Can you work these out from the model? Positions are in its coordinate system, mm. A direction names the side the tool comes from. Coordinates: 2 decimals unless noted, no trailing zeros. Order: outer loops, then holes, each group sorted by start corner. A loop starts at its lowest first (then second) coordinate and runs counter-clockwise, first axis right, second up. Notation, with made-up numbers: (78.25, 17.25) - (92.25, 17.25) arc R18 ccw to (92.25, 25.25) - close; hole circle Ø1 at (57.5, 9.5). An arc over 180 degrees is marked (long way). Use a Markdown table: item, result. Add a question column.
(1) I want a section at D-D (z = -5.5). List the corners of the cut face in (x, y) for me.
(2) I want a section at B-B (y = 0). List the corners of the cut face in (x, z) for me, and give its area (3 significant figures).
(3) We'd pull the mould along X, two halves only. Please class faces 1 (the cylindrical face through (-13.976, 14.868, 23.171)), 2 (the flat face through (-18.6, -18.7, 23.2)), 3 (the flat face through (3, 0, -2)): pulls with the +X half, pulls with the -X half, needs draft (parallel to the pull), parting line crosses it, or undercut.
(4) I want a section at A-A (z = 18). List the corners of the cut face in (x, y) for me, and give its area (3 significant figures).
(5) If I drill on L1, parallel to Y at x = -15.5, z = 29.5; L2, parallel to Z at x = 4, y = -8; L3, parallel to Z at x = -4, y = 11, over which ranges is the centre line in solid material (lowest first)? Write a range as [from, to].
(6) I want a section at C-C (x = 0). List the corners of the cut face in (y, z) for me, and give its area (3 significant figures).
(7) On a 3-axis mill with a long thin cutter (end or side, diameter ignored), from which of +Z, -Z, +X, -X, +Y, -Y can I reach the whole of each face in a straight line? I mean faces 4 (the cylindrical face through (17.024, 14.868, 23.171)), 5 (the cylindrical face through (-0.1, -2.5, -7.9)), 6 (the flat face through (0, 2, -8)). Say none if no direction works.
(8) For pin 1 Ø21 at (x, y) = (-3, -8) entering from -Z; pin 2 Ø0.9 at (x, z) = (0.5, -8) entering from +Y; pin 3 Ø3 at (x, z) = (-5, -4.5) entering from -Y; pin 4 Ø4 at (x, y) = (15.5, -15.5) entering from -Z, each with a flat end and sliding along its axis, tell me the tip position at first contact or that it passes through.
```python
from build123d import *

# Parameters (mm, degrees)
SKETCH_1_R          = 1.65
EXTRUDE_1_DEPTH     = 47
SKETCH_3_R          = 11
EXTRUDE_2_DEPTH     = 2
EXTRUDE_3_DEPTH     = 22
CUT_EXTRUDE_1_DEPTH = 10


with BuildPart() as part:
    # 草图1 → 凸台-拉伸1 (new body)
    with BuildSketch(Plane.XY):
        Polygon((-21.15, 16.15), (-16.15, 21.15), (16.15, 21.15), (21.15, 16.15), (21.15, -16.15), (16.15, -21.15), (-16.15, -21.15), (-21.15, -16.15), align=None)
        with Locations((15.5, 15.5)):
            Circle(SKETCH_1_R, mode=Mode.SUBTRACT)
        with Locations((-15.5, 15.5)):
            Circle(SKETCH_1_R, mode=Mode.SUBTRACT)
        with Locations((15.5, -15.5)):
            Circle(SKETCH_1_R, mode=Mode.SUBTRACT)
        with Locations((-15.5, -15.5)):
            Circle(SKETCH_1_R, mode=Mode.SUBTRACT)
    extrude(amount=EXTRUDE_1_DEPTH)

    # 草图3 → 凸台-拉伸2 (add)
    with BuildSketch(Plane(origin=(0, 0, 0), x_dir=(-1, 0, 0), z_dir=(0, 0, -1))):
        Circle(SKETCH_3_R)
    extrude(amount=EXTRUDE_2_DEPTH)

    # 草图4 → 凸台-拉伸3 (add)
    with BuildSketch(Plane(origin=(0, 0, -2), x_dir=(-1, 0, 0), z_dir=(0, 0, -1))):
        with BuildLine():
            Line((-1.5, 2), (1.5, 2))
            ThreePointArc((1.5, 2), (0, -2.5), (-1.5, 2))
        make_face()
    extrude(amount=EXTRUDE_3_DEPTH)

    # 草图5 → 切除-拉伸1 (cut)
    with BuildSketch(Plane(origin=(0, 0, -24), x_dir=(-1, 0, 0), z_dir=(0, 0, -1))):
        with BuildLine():
            Line((1.5, 2), (-1.5, 2))
            ThreePointArc((-1.5, 2), (0, -2.5), (1.5, 2))
        make_face()
    extrude(amount=-CUT_EXTRUDE_1_DEPTH, mode=Mode.SUBTRACT)


solid = part.part
```
Answers follow:
| question | item | result |
|---|---|---|
| 1 | outline | (-1.5, 2) arc R2.5 ccw (long way) to (1.5, 2) - close |
| 2 | outline | (-21.15, 0) - (-11, 0) - (-11, -2) - (-2.5, -2) - (-2.5, -14) - (2.5, -14) - (2.5, -2) - (11, -2) - (11, 0) - (21.15, 0) - (21.15, 47) - (-21.15, 47) - close |
| 2 | area | 2,090 mm² |
| 3 | face 1 | undercut |
| 3 | face 2 | pulls with the -X half |
| 3 | face 3 | needs draft |
| 4 | outline | (-21.15, -16.15) - (-16.15, -21.15) - (16.15, -21.15) - (21.15, -16.15) - (21.15, 16.15) - (16.15, 21.15) - (-16.15, 21.15) - (-21.15, 16.15) - close; hole circle Ø3.3 at (-15.5, -15.5); hole circle Ø3.3 at (-15.5, 15.5); hole circle Ø3.3 at (15.5, -15.5); hole circle Ø3.3 at (15.5, 15.5) |
| 4 | area | 1,710 mm² |
| 5 | L1 | y = [-21.15, -17.15], [-13.85, 13.85], [17.15, 21.15] |
| 5 | L2 | z = [-2, 47] |
| 5 | L3 | z = [0, 47] |
| 6 | outline | (-21.15, 0) - (-11, 0) - (-11, -2) - (-2.5, -2) - (-2.5, -14) - (2, -14) - (2, -2) - (11, -2) - (11, 0) - (21.15, 0) - (21.15, 47) - (-21.15, 47) - close |
| 6 | area | 2,090 mm² |
| 7 | face 4 | +Z, -Z |
| 7 | face 5 | -Z |
| 7 | face 6 | -Z, +X, -X, +Y |
| 8 | pin 1 | stops at z = -14 |
| 8 | pin 2 | stops at y = 2 |
| 8 | pin 3 | passes through |
| 8 | pin 4 | stops at z = 0 |
